```python
from build123d import *

# Parameters (mm, degrees)
SKETCH1_R                 = 12.5
BOSS_EXTRUDE1_DEPTH       = 115
CHAMFER1_SIZE             = 2
BOSS_EXTRUDE2_DEPTH       = 10
F_8_0MM_DOWEL_HOLE1_D     = 8.5
F_8_0MM_DOWEL_HOLE1_DEPTH = 70
F_8_0MM_DOWEL_HOLE1_TIP   = 2.553657631
CUT_EXTRUDE1_START        = -13
SKETCH7_R                 = 5
SKETCH7_R_2               = 4.25
CUT_EXTRUDE1_DEPTH        = 13
CUT_EXTRUDE2_DEPTH        = 129.317659161
CUT_EXTRUDE2_DEPTH_BACK   = 129.317659161
SKETCH10_R                = 4.25
SKETCH11_W                = 1.5
SKETCH11_H                = 4.762269722
CHAMFER2_SIZE             = 0.3
CHAMFER3_SIZE             = 0.3


with BuildPart() as part:
    # Sketch1 → Boss-Extrude1 (new body)
    with BuildSketch(Plane(origin=(0, 0, 0), x_dir=(0, 0, -1), z_dir=(1, 0, 0))):
        Circle(SKETCH1_R)
    extrude(amount=BOSS_EXTRUDE1_DEPTH)

    # Chamfer1
    chamfer1_edges = [part.edges().sort_by_distance(p)[0] for p in [
        (0, 0, 12.5),
    ]]
    chamfer(chamfer1_edges, length=CHAMFER1_SIZE)

    # Sketch3 → Boss-Extrude2 (add)
    with BuildSketch(Plane(origin=(115, 0, 0), x_dir=(0, 0, -1), z_dir=(1, 0, 0))):
        Polygon((11.093502405, -18.847185944), (21.86889302, 0.183661927), (10.775390615, 19.030847871), (-11.093502405, 18.847185944), (-21.86889302, -0.183661927), (-10.775390615, -19.030847871), align=None)
    extrude(amount=BOSS_EXTRUDE2_DEPTH)

    # Ø8.0mm Dowel Hole1
    with Locations(Plane(origin=(125, 0, 0), x_dir=(0, 0, -1), z_dir=(1, 0, 0))):
        with Locations((0, 0)):
            Hole(F_8_0MM_DOWEL_HOLE1_D / 2, depth=F_8_0MM_DOWEL_HOLE1_DEPTH)
            with Locations((0, 0, -(F_8_0MM_DOWEL_HOLE1_DEPTH + F_8_0MM_DOWEL_HOLE1_TIP / 2))):  # 118° drill point
                Cone(0, F_8_0MM_DOWEL_HOLE1_D / 2, F_8_0MM_DOWEL_HOLE1_TIP, mode=Mode.SUBTRACT)

    # Sketch7 → Cut-Extrude1 (cut)
    with BuildSketch(Plane(origin=(125, 0, 0), x_dir=(0, 0, -1), z_dir=(1, 0, 0)).offset(CUT_EXTRUDE1_START)):
        Circle(SKETCH7_R)
        Circle(SKETCH7_R_2, mode=Mode.SUBTRACT)
    extrude(amount=CUT_EXTRUDE1_DEPTH, mode=Mode.SUBTRACT)

    # Sketch10 → Cut-Extrude2 (cut, two sides: drawn at the far end of the back side and taken through both)
    with BuildSketch(Plane(origin=(0, 0, 0), x_dir=(1, 0, 0), z_dir=(0, 1, 0)).offset(-CUT_EXTRUDE2_DEPTH_BACK)):
        with Locations(Location((64, 0, 0), (0, 0, 270))):
            Circle(SKETCH10_R)
    extrude(amount=CUT_EXTRUDE2_DEPTH + CUT_EXTRUDE2_DEPTH_BACK, mode=Mode.SUBTRACT)

    # Sketch11 → Cut-Revolve3 (revolve, cut)
    with BuildSketch(Plane.XY, mode=Mode.PRIVATE) as cut_revolve3_sk:
        with Locations((12.25, 14.506134861)):
            Rectangle(SKETCH11_W, SKETCH11_H)
    revolve(cut_revolve3_sk.sketch.rotate(Axis((-5.779414499, 0, 0), (1, 0, 0)), 270), axis=Axis((-5.779414499, 0, 0), (1, 0, 0)), mode=Mode.SUBTRACT)

    # Chamfer2
    chamfer2_edges = [part.edges().sort_by_distance(p)[0] for p in [
        (13, 0, 12.5),
    ]]
    chamfer(chamfer2_edges, length=CHAMFER2_SIZE)

    # Chamfer3
    chamfer3_edges = [part.edges().sort_by_distance(p)[0] for p in [
        (11.5, 0, 12.5),
    ]]
    chamfer(chamfer3_edges, length=CHAMFER3_SIZE)


solid = part.part
```
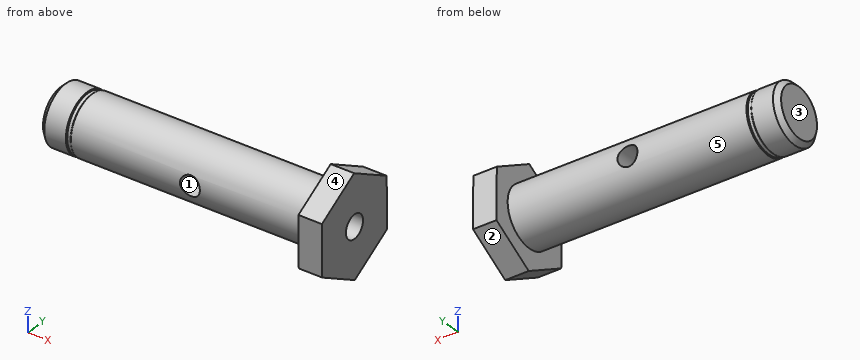
Can you work these out from the model? Positions are in its coordinate system, mm. Face numbers are marked on the shaded views. A direction names the side the tool comes from. Give positions to 0.01 mm unless a question says otherwise; leave off trailing zeros. Write each loop counter-clockwise with the first axis right and the second up, starting at its lowest first coordinate (ties: lowest second). Pieces come first, ordered by that corner, then holes. Notation, with made-up numbers: (79, -39.75) - (87, -39.75) arc R10 ccw to (87, -30.75) - close; hole circle Ø5 at (72, 2). An arc over 180 degrees is marked (long way). Write item = value, one per line. Start each with the question number.
1. Imagine slicing it at A-A (x = 66.5). Please give me the cut outline in (y, z).
2. For pin 1 (1.5 mm diameter, centred on y = 12, z = -16.5, fed in from +X); pin 2 (3 mm diameter, centred on y = 1.5, z = -1.5, fed in from +X); pin 3 (2 mm diameter, centred on x = 59, y = 2.5, fed in from +Z); pin 4 (10 mm diameter, centred on x = 57.5, z = -11, fed in from -Y), each with a flat end and sliding along its axis, tell me the tip position at first contact or that it passes through.
3. On a 3-axis mill with a long thin cutter (end or side, diameter ignored), from which of +Z, -Z, +X, -X, +Y, -Y can I reach the whole of each face in a straight line? I mean the marked faces 4 and 5. Say none if no direction works.
4. Imagine slicing it at C-C (z = -3). Count the separate pieces of the cut face and the enclosed holes in it, and give its area (3 significant figures).
5. Please list where these lines run through material, in increasing order: line 1 (X direction, y = -5.75, z = 0); line 2 (X direction, y = -12, z = -9); line 3 (X direction, y = -9.5, z = -1.5).
6. Imagine slicing it at B-B (x = 94.5). Please give me the cut outline in (y, z).
7. Thinking about a two-plate mould opening in X: for the marked faces 1, 2 and 3, which applies, released by +X, released by -X, zero draft, split by the parting line, or undercut?
8. Imagine slicing it at D-D (x = 27.5). Please give me the cut outline in (y, z), and give its area (3 significant figures).
Worked answers:
q1.outline = (-12.02, -3.44) arc R12.5 ccw to (12.02, -3.44) - (2.5, -3.44) arc R4.25 cw to (-2.5, -3.44) - close; (-12.02, 3.44) - (-2.5, 3.44) arc R4.25 cw to (2.5, 3.44) - (12.02, 3.44) arc R12.5 ccw to start
q2.pin_1 = through
q2.pin_2 = 54.62
q2.pin_3 = 12.41
q2.pin_4 = -10.97
q3.face_4 = +Z, +X, -X, -Y
q3.face_5 = -X
q4.separate_pieces = 3
q4.enclosed_holes = 0
q4.area = 2,600 mm2
q5.line_1 = 0 to 59.75, 68.25 to 125
q5.line_2 = 115 to 125
q5.line_3 = 0 to 60.02, 67.98 to 125
q6.outline = circle Ø25 at (0, 0); hole circle Ø8.5 at (0, 0)
q7.face_1 = undercut
q7.face_2 = zero draft
q7.face_3 = released by -X
q8.outline = circle Ø25 at (0, 0)
q8.area = 491 mm2
